Part model, mm, in its own coordinate system. Face numbers are marked on the shaded views. A direction names the side the tool comes from. Give positions to 0.01 mm unless a question says otherwise; leave off trailing zeros. Write each loop counter-clockwise with the first axis right and the second up, starting at its lowest first coordinate (ties: lowest second). Pieces come first, ordered by that corner, then holes. Notation, with made-up numbers: M 34,54 L 88,54 A13 ccw 88,72 Z; hole C -37,79 d5. An arc over 180 degrees is marked long. Use CSV: the item, a comma, the result in double quotes. Start each with the question number.
1. Band-saw the part on C-C, the plane x = 8. List the corners of the cut face in (y, z).
2. Mould opens along Y. For the marked faces 1, 2 and 3 say: pulls with the +Y half, pulls with the -Y half, needs draft (parallel to the pull), parting line crosses it, or undercut.
3. Drill centre lines: line 1 along X through (y, z) = (-1.5, 4); line 2 along X through (y, z) = (0, 22); line 3 along Y through (x, z) = (-46, 27). Where is each one in solid material? Low to high. Write a range as from..to.
4. Drop flat-ended pins along their axis: pin 1 Ø3 at (x, z) = (2, 14.5) entering from -Y; pin 2 Ø1.5 at (y, z) = (4.5, 18.5) entering from -X; pin 3 Ø4 at (x, y) = (-32.5, 0) entering from +Z; pin 4 Ø1.3 at (x, z) = (-31.5, 14) entering from +Y. Give the stop position or say it passes through.
5. Band-saw the part on B-B, the plane z = 7.5. Count the separate pieces of the cut face and the enclosed holes in it, then the cut area to 3 significant figures.
6. 3-axis set-ups, long thin cutter, end or side, ignore diameter. For the marked faces 4 and 5: which of +Z, -Z, +X, -X, +Y, -Y reach the whole face in a straight line?
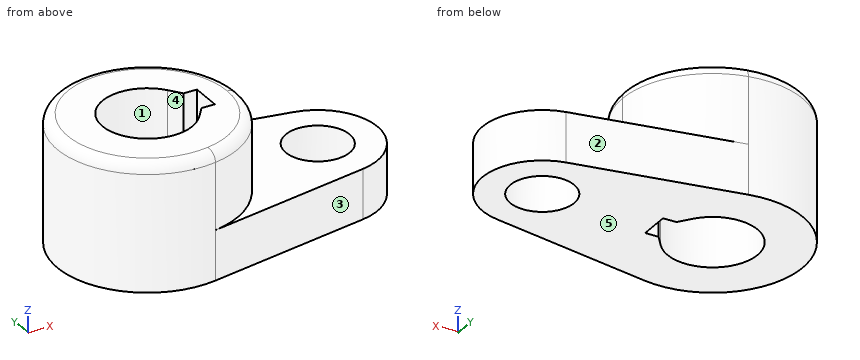
from build123d import *

# Parameters (mm, degrees)
F0_R     = 10.16
F1_DEPTH = 15.7734
F2_DEPTH = 40.2336
F3_R     = 3.302


with BuildPart() as f1:
    # F0 (on Top) → F1 (new body)
    with BuildSketch(Plane.XY):
        with BuildLine():
            ThreePointArc((-42.744664, 28.116476), (-25.908921, 18.3145), (-19.268134, 0))
            ThreePointArc((-19.268134, 0), (-25.908921, -18.3145), (-42.744664, -28.116476))
            Line((-42.744664, -28.116476), (9.512032, -18.640565))
            ThreePointArc((9.512032, -18.640565), (25.076422, 0), (9.512032, 18.640565))
            Line((9.512032, 18.640565), (-42.744664, 28.116476))
        make_face()
        with Locations((6.131866, 0)):
            Circle(F0_R, mode=Mode.SUBTRACT)
    extrude(amount=F1_DEPTH)

    # F0 (on Top) → F2 (join)
    with BuildSketch(Plane.XY):
        with BuildLine():
            ThreePointArc((-42.744664, -28.116476), (-25.908921, -18.3145), (-19.268134, 0))
            ThreePointArc((-19.268134, 0), (-25.908921, 18.3145), (-42.744664, 28.116476))
            ThreePointArc((-42.744664, 28.116476), (-76.418134, 0), (-42.744664, -28.116476))
        make_face()
        with BuildLine():
            ThreePointArc((-36.481987, -8.663543), (-62.130634, 0), (-36.481987, 8.663543))
            Line((-36.481987, 8.663543), (-33.555634, 4.826))
            Line((-33.555634, 4.826), (-29.313834, 4.826))
            Line((-29.313834, 4.826), (-29.313834, 0))
            Line((-29.313834, 0), (-29.313834, -4.826))
            Line((-29.313834, -4.826), (-33.555634, -4.826))
            Line((-33.555634, -4.826), (-36.481987, -8.663543))
        make_face(mode=Mode.SUBTRACT)
    extrude(amount=F2_DEPTH)

    # F3
    f3_edges = [f1.edges().sort_by_distance(p)[0] for p in [
        (-52.941605, 28.116476, 40.2336),
    ]]
    fillet(f3_edges, radius=F3_R)


solid = f1.part
Output:
1,outline,"M -18.91,0 L -9.99,0 L -9.99,15.77 L -18.91,15.77 Z; M 9.99,0 L 18.91,0 L 18.91,15.77 L 9.99,15.77 Z"
2,face 1,"undercut"
2,face 2,"pulls with the +Y half"
2,face 3,"pulls with the -Y half"
3,line 1,"x = -76.38..-62.05, -29.31..-3.92, 16.18..25.02"
3,line 2,"x = -76.42..-62.13, -29.31..-19.27"
3,line 3,"y = -28.52..-14.17, 14.17..28.52"
4,pin 1,"stops at y = -20.27"
4,pin 2,"stops at x = -76.17"
4,pin 3,"passes through"
4,pin 4,"stops at y = 26.2"
5,separate pieces,"1"
5,enclosed holes,"2"
5,area,"3,440 mm²"
6,face 4,"+Z, -Z"
6,face 5,"-Z, +X, -X, +Y, -Y"
